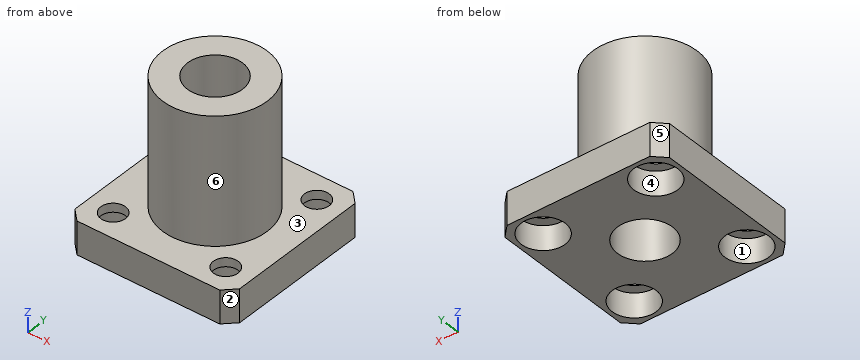
```python
from build123d import *

# Parameters (mm, degrees)
SKETCH1_W                               = 30
SKETCH1_H                               = 30
BOSS_EXTRUDE1_DEPTH                     = 6
SKETCH2_R                               = 9.5
BOSS_EXTRUDE2_DEPTH                     = 23
SKETCH3_R                               = 5
CUT_EXTRUDE1_DEPTH                      = 52.39066063
CBORE_FOR_M5_HEX_HEAD_BOLT1_D           = 4.5
CBORE_FOR_M5_HEX_HEAD_BOLT1_CBORE_D     = 8
CBORE_FOR_M5_HEX_HEAD_BOLT1_CBORE_DEPTH = 4.4
CHAMFER1_SIZE                           = 2


with BuildPart() as part:
    # Sketch1 → Boss-Extrude1 (new body)
    with BuildSketch(Plane.XY):
        with Locations((15, 15)):
            Rectangle(SKETCH1_W, SKETCH1_H)
    extrude(amount=BOSS_EXTRUDE1_DEPTH)

    # Sketch2 → Boss-Extrude2 (add)
    with BuildSketch(Plane.XY.offset(6)):
        with Locations((15, 15)):
            Circle(SKETCH2_R)
    extrude(amount=BOSS_EXTRUDE2_DEPTH)

    # Sketch3 → Cut-Extrude1 (cut, through all)
    with BuildSketch(Plane.XY.offset(29)):
        with Locations((15, 15)):
            Circle(SKETCH3_R)
    extrude(amount=-CUT_EXTRUDE1_DEPTH, mode=Mode.SUBTRACT)

    # CBORE for M5 Hex Head Bolt1 (through all)
    with Locations(Plane(origin=(0, 0, 0), x_dir=(-1, 0, 0), z_dir=(0, 0, -1))):
        with Locations((-25.253048327, 25.253048327), (-4.746951673, 25.253048327), (-4.746951673, 4.746951673), (-25.253048327, 4.746951673)):
            CounterBoreHole(CBORE_FOR_M5_HEX_HEAD_BOLT1_D / 2, CBORE_FOR_M5_HEX_HEAD_BOLT1_CBORE_D / 2, CBORE_FOR_M5_HEX_HEAD_BOLT1_CBORE_DEPTH)

    # Chamfer1
    chamfer1_edges = [part.edges().sort_by_distance(p)[0] for p in [
        (0, 30, 3),
        (30, 30, 3),
        (30, 0, 3),
        (0, 0, 3),
    ]]
    chamfer(chamfer1_edges, length=CHAMFER1_SIZE)


solid = part.part
```
Geometry check sheet. Reference: the model listing, model coordinates, mm. Face numbers are marked on the shaded views. A direction names the side the tool comes from. Round coordinates to 2 decimals unless told otherwise and drop trailing zeros. Loops run counter-clockwise (first coordinate to the right, second up) from the corner with the lowest first, then second, coordinate; pieces in that order, holes last. Notation, with made-up numbers: (63, -22) -> (101, -22) arc R14 cw to (101, -15) -> close; hole circle Ø1 at (71, -15). An arc over 180 degrees is marked (long way). Use a Markdown table: item, result.
(1) Sectioned sample at B-B (y = 15). Enter the section's corners in (x, z).
Calculated:
| item | result |
|---|---|
| outline | (0, 0) -> (10, 0) -> (10, 29) -> (5.5, 29) -> (5.5, 6) -> (0, 6) -> close; (20, 0) -> (30, 0) -> (30, 6) -> (24.5, 6) -> (24.5, 29) -> (20, 29) -> close |
(2) Scan lines: probe 1 along X at (y, z) = (25, 1.75); probe 2 along Z at (x, y) = (8.5, 3.75); probe 3 along Z at (x, y) = (12.75, 25.75). Record each from-to range of solid material in increasing order.
Calculated:
| item | result |
|---|---|
| probe 1 | 0 to 0.75, 8.74 to 21.26, 29.25 to 30 |
| probe 2 | 4.4 to 6 |
| probe 3 | 0 to 6 |
(3) Sectioned sample at A-A (x = 25.25). Enter the section's corners in (y, z), then the cut area to 3 significant figures.
Calculated:
| item | result |
|---|---|
| outline | (0, 0) -> (0.75, 0) -> (0.75, 4.4) -> (2.5, 4.4) -> (2.5, 6) -> (0, 6) -> close; (7, 4.4) -> (8.75, 4.4) -> (8.75, 0) -> (21.25, 0) -> (21.25, 4.4) -> (23, 4.4) -> (23, 6) -> (7, 6) -> close; (27.5, 4.4) -> (29.25, 4.4) -> (29.25, 0) -> (30, 0) -> (30, 6) -> (27.5, 6) -> close |
| area | 95.2 mm² |
(4) Go/stop test with flat-tipped pins: P1, Ø12, axis at x = 15, z = 21, coming from the -Y side; P2, Ø2, axis at y = 7, z = 9, coming from the -X side; P3, Ø7, axis at x = 25.25, y = 4.75, coming from the -Z side; P4, Ø3.5, axis at x = 4.75, y = 25.25, coming from the -Z side. Record where each tip stops, or that it passes through.
Calculated:
| item | result |
|---|---|
| P1 | y = 5.5 |
| P2 | x = 8.58 |
| P3 | z = 4.4 |
| P4 | through |
(5) Mould release check, pull along Y, two halves, no side actions. Record for the marked faces 1, 2 and 3: released by +Y, released by -Y, zero draft, split by the parting line, or undercut.
Calculated:
| item | result |
|---|---|
| face 1 | undercut |
| face 2 | released by -Y |
| face 3 | zero draft |
(6) Set-up check for the marked faces 4, 5 and 6: record each of +Z, -Z, +X, -X, +Y, -Y from which the full face is reachable in a straight line by a thin tool's end or side.
Calculated:
| item | result |
|---|---|
| face 4 | -Z |
| face 5 | +Z, -Z, -X, +Y |
| face 6 | +Z |
(7) Sectioned sample at D-D (z = 23.25). Enter the section's corners in (x, y).
Calculated:
| item | result |
|---|---|
| outline | circle Ø19 at (15, 15); hole circle Ø10 at (15, 15) |
